For this review, take the finished solid that the model builds, in its own axes (mm). A direction names the side the tool comes from. Give positions to 0.01 mm unless a question says otherwise; leave off trailing zeros. Order: outer loops, then holes, each group sorted by start corner. A loop starts at its lowest first (then second) coordinate and runs counter-clockwise, first axis right, second up. Notation, with made-up numbers: M 79,75.25 L 97,75.25 A28 cw 97,112.25 Z; hole C 87.5,-5 d6. An arc over 180 degrees is marked long. Use CSV: the item, a comma, the result in double quotes. Start each with the question number.
(1) Wall thickness on L1, parallel to Z at x = 23.5, y = 30.5; L2, parallel to Y at x = -6, z = 38.5; L3, parallel to Y at x = -20.5, z = 28: over which ranges is each line inside the solid? List them lowest first. Write a range as from..to.
(2) Consider section A-A (y = -28.5). Write out the cut boundary in (x, z), and give its area (3 significant figures).
(3) Consider section B-B (x = -8). Write out the cut boundary in (y, z).
(4) Tool access review of faces 4 (the face through (7, -39.688, 25)), 5 (the face through (-22, -22, 19.05)), 6 (the face through (0, 30, 38.1)): name each direction out of +Z, -Z, +X, -X, +Y, -Y from which nothing blocks a thin tool from reaching the whole face with its end or side.
(5) Clearance check with flat-ended pins moving along their axes: P1, Ø6.5, axis at x = -7.5, z = 43.5, coming from the +Y side; P2, Ø11, axis at x = -25.5, y = -28, coming from the +Z side; P3, Ø18, axis at x = -21.5, z = 31, coming from the -Y side. State where each tip first meets the part, or that it passes through.
(6) Draft analysis for pull direction Y (two halves, no side actions). For faces 1 (the face through (-22, -4.763, 35)), 2 (the face through (-33.338, 8, 19)), 3 (the face through (0, 39.688, 19)), state which applies: pulls with the +Y half, pulls with the -Y half, needs draft (parallel to the pull), parting line crosses it, or undercut.
```python
from build123d import *

# Parameters (mm, degrees)
F0_W     = 66.675
F0_H     = 79.375
F1_DEPTH = 50.8
F2_W     = 66.675
F2_H     = 19.05
F3_DEPTH = 12.7
F4_W     = 22.225
F4_H     = 34.925
F5_DEPTH = 31.75


with BuildPart() as f1:
    # F0 (on Top) → F1 (new body)
    with BuildSketch(Plane.XY):
        Rectangle(F0_W, F0_H)
    extrude(amount=F1_DEPTH)

    # F2 (on face) → F3 (cut)
    with BuildSketch(Plane.XY.offset(50.8)):
        with Locations((0, 30.1625)):
            Rectangle(F2_W, F2_H)
    extrude(amount=-F3_DEPTH, mode=Mode.SUBTRACT)

    # F4 (on face) → F5 (cut)
    with BuildSketch(Plane.XY.offset(50.8)):
        with Locations((-22.225, -22.225)):
            Rectangle(F4_W, F4_H)
    extrude(amount=-F5_DEPTH, mode=Mode.SUBTRACT)


solid = f1.part
```
Check result:
1,L1,"z = 0..38.1"
1,L2,"y = -39.69..20.64"
1,L3,"y = -4.76..39.69"
2,outline,"M -33.34,0 L 33.34,0 L 33.34,50.8 L -11.11,50.8 L -11.11,19.05 L -33.34,19.05 Z"
2,area,"2,680 mm^2"
3,outline,"M -39.69,0 L 39.69,0 L 39.69,38.1 L 20.64,38.1 L 20.64,50.8 L -39.69,50.8 Z"
4,face 4,"+Z, -Z, +X, -X, -Y"
4,face 5,"+Z, -X, -Y"
4,face 6,"+Z, +X, -X, +Y"
5,P1,"stops at y = 20.64"
5,P2,"stops at z = 19.05"
5,P3,"stops at y = -4.76"
6,face 1,"pulls with the -Y half"
6,face 2,"needs draft"
6,face 3,"pulls with the +Y half"
